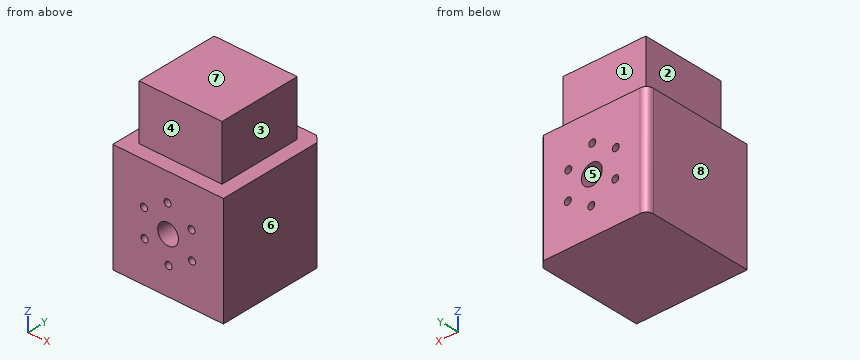
Autodesk Inventor part; units mm, degrees
ref_plane "YZ Plane" through (0, 0, 0) normal (1, 0, 0) x (0, 1, 0)
ref_plane "XZ Plane" through (0, 0, 0) normal (0, 1, 0) x (-1, 0, 0)
ref_plane "XY Plane" through (0, 0, 0) normal (0, 0, 1) x (1, 0, 0)
sketch "Sketch1" plane through (0, 0, 0) normal (0, 1, 0) x (-1, 0, 0)
  line L0 (0, 0) -> (101.6, 0)
  line L1 (101.6, 0) -> (101.6, -101.6)
  line L2 (101.6, -101.6) -> (0, -101.6)
  line L3 (0, -101.6) -> (0, 0)
  dimension "d0" = 101.6
  dimension "d1" = 101.6
extrude "Extrusion1" add sketch "Sketch1" along normal blind 101.6
sketch "Sketch2" plane through (0, 101.6, 0) normal (0, 1, 0) x (1, 0, 0)
  circle A0 centre (-50.8, 50.8) radius 9.525
  line L0 (-101.6, 0) -> (0, 0)
  line L1 (-101.6, 101.6) -> (-101.6, 0)
  point P0 (-51.2601, 25.6301)
  point P1 (-29.2322, 37.8166)
  point P2 (-28.7721, 62.9865)
  point P3 (-50.3399, 75.9699)
  point P4 (-72.3678, 63.7834)
  point P5 (-72.8279, 38.6135)
  dimension "d6" = 360
  dimension "d25" = 19.05
  dimension "d26" = 50.8
  dimension "d27" = 50.8
extrude "Extrusion2" cut sketch "Sketch2" against normal through all
hole "Hole1" at (-50.8, 101.6, -50.8) at (-51.2601, 101.6, -25.6301) at (-29.2322, 101.6, -37.8166) at (-28.7721, 101.6, -62.9865) at (-50.3399, 101.6, -75.9699) at (-72.3678, 101.6, -63.7834) at (-72.8279, 101.6, -38.6135) direction (0, -1, 0) diameter 6.35 end through all
fillet "Fillet1" radius 6.35 1 edges at (-101.6, 101.6, -50.8)
chamfer "Chamfer1" distance 6.35 angle 45 1 edges at (0, 101.6, -50.8)
sketch "Sketch3" plane through (-101.6, 0, 0) normal (0, 0, 1) x (1, 0, 0)
  line L0 (12.7, 88.9) -> (88.9, 88.9)
  line L1 (88.9, 88.9) -> (88.9, 12.7)
  line L2 (88.9, 12.7) -> (12.7, 12.7)
  line L3 (12.7, 12.7) -> (12.7, 88.9)
  line L4 (12.7, 88.9) -> (88.9, 12.7) construction
  line L5 (88.9, 88.9) -> (12.7, 12.7) construction
  point P0 (101.6, 0)
  point P1 (50.8, 50.8)
  dimension "d21" = 76.2
  dimension "d22" = 76.2
extrude "Extrusion3" add sketch "Sketch3" along normal blind 50.8
properties part number "BasicCube"
Verification items for the finished model (mm, model axes). Face numbers are marked on the shaded views. A direction names the side the tool comes from. Give positions to 0.01 mm unless a question says otherwise; leave off trailing zeros. Order: outer loops, then holes, each group sorted by start corner. A loop starts at its lowest first (then second) coordinate and runs counter-clockwise, first axis right, second up. Notation, with made-up numbers: M -34.75,65 L 7.25,65 A15 ccw 7.25,70 Z; hole C 9.5,-16.75 d4. An arc over 180 degrees is marked long. Answer in a Markdown table with one row per item. Add a question column.
Item 1: Section check C-C, the plane y = 86. State how many separate pieces and enclosed holes the cut face has, and give its area (3 significant figures).
Item 2: Tool access check on the marked faces 1, 2, 3 and 4. Record the directions out of +Z, -Z, +X, -X, +Y, -Y that give a thin tool (end or side, any length) a straight path to the whole face; none if there is none.
Item 3: Gauge pin test, flat ends, axial feed: pin 1 (4 mm diameter, centred on x = -72.37, z = -63.78, fed in from -Y); pin 2 (5 mm diameter, centred on x = -73.5, z = 5, fed in from -Y); pin 3 (1 mm diameter, centred on x = -68.5, z = 10, fed in from +Y). Record the tip position at first contact, or that the pin passes through.
Item 4: Scan lines: probe 1 along Z at (x, y) = (-29, 26.5); probe 2 along Z at (x, y) = (-28, 9); probe 3 along Z at (x, y) = (-11.5, 7). Record each from-to range of solid material in increasing order. Write a range as from..to.
Item 5: Section check B-B, the plane x = -84. Enter the section's corners in (y, z), and give its area (3 significant figures).
Item 6: Mould release check, pull along X, two halves, no side actions. Record for the marked faces 5, 6, 7 and 8: released by +X, released by -X, zero draft, split by the parting line, or undercut.
Item 7: Section check A-A, the plane z = -50.8. Enter the section's corners in (x, y) (3 decimals).
Filled sheet:
| question | item | result |
|---|---|---|
| 1 | separate pieces | 1 |
| 1 | enclosed holes | 7 |
| 1 | area | 13,700 mm^2 |
| 2 | face 1 | +Z, +X, -X, +Y |
| 2 | face 2 | +Z, -X, +Y, -Y |
| 2 | face 3 | +Z, +X, +Y, -Y |
| 2 | face 4 | +Z, +X, -X, -Y |
| 3 | pin 1 | passes through |
| 3 | pin 2 | stops at y = 12.7 |
| 3 | pin 3 | stops at y = 88.9 |
| 4 | probe 1 | z = -101.6..-66.15, -59.82..-40.98, -34.65..50.8 |
| 4 | probe 2 | z = -101.6..-66.07, -59.91..-40.74, -34.89..0 |
| 4 | probe 3 | z = -101.6..0 |
| 5 | outline | M 0,-101.6 L 101.6,-101.6 L 101.6,0 L 88.9,0 L 88.9,50.8 L 12.7,50.8 L 12.7,0 L 0,0 Z |
| 5 | area | 14,200 mm^2 |
| 6 | face 5 | undercut |
| 6 | face 6 | released by +X |
| 6 | face 7 | zero draft |
| 6 | face 8 | released by -X |
| 7 | outline | M -101.6,0 L -60.325,0 L -60.325,101.6 L -95.25,101.6 A6.35 ccw -101.6,95.25 Z; M -41.275,0 L 0,0 L 0,95.25 L -6.35,101.6 L -41.275,101.6 Z |
